Build history of the part. All positions in model axes, mm. Coordinates: 2 decimals unless noted, no trailing zeros. Loops run counter-clockwise (first coordinate to the right, second up) from the corner with the lowest first, then second, coordinate; pieces in that order, holes last. Notation, with made-up numbers: (21.5, 26.5) - (65.5, 26.5) arc R9 cw to (65.5, 40.5) - close; hole circle Ø7 at (-28, 86). An arc over 180 degrees is marked (long way). One line per item, written item: value.
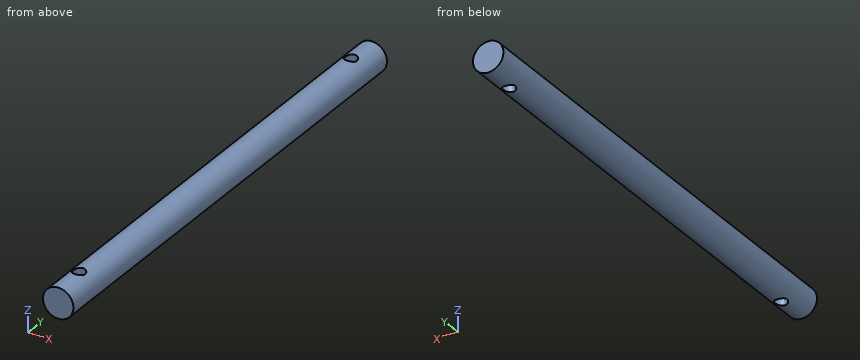
```python
from build123d import *

# Parameters (mm, degrees)
SKETCH1_R           = 3.96
BOSS_EXTRUDE1_DEPTH = 65.09
SKETCH2_R           = 1.59
CUT_EXTRUDE1_DEPTH  = 66.330477574


with BuildPart() as part:
    # Sketch1 → Boss-Extrude1 (new, symmetric)
    with BuildSketch(Plane(origin=(0, 0, 0), x_dir=(1, 0, 0), z_dir=(0, 1, 0))):
        with Locations(Location((0, 0, 0), (0, 0, 270))):
            Circle(SKETCH1_R)
    extrude(amount=BOSS_EXTRUDE1_DEPTH, both=True)

    # Sketch2 → Cut-Extrude1 (cut, symmetric)
    with BuildSketch(Plane.XY):
        with Locations(Location((0, 56.43, 0), (0, 0, 90))):
            Circle(SKETCH2_R)
    cut_extrude1 = extrude(amount=CUT_EXTRUDE1_DEPTH, both=True, mode=Mode.SUBTRACT)

    # Mirror1: Cut-Extrude1 across plane
    add(cut_extrude1.mirror(Plane.ZX), mode=Mode.SUBTRACT)


solid = part.part
```
Item 1: Cut at B-B, the plane z = 0. Write the cut outline in (x, y).
Check result:
outline: (-3.96, -65.09) - (3.96, -65.09) - (3.96, 65.09) - (-3.96, 65.09) - close; hole circle Ø3.18 at (0, -56.43); hole circle Ø3.18 at (0, 56.43)
Item 2: Cut at C-C, the plane y = 52. Write the cut outline in (x, z), then the cut area to 3 significant figures.
Check result:
outline: circle Ø7.92 at (0, 0)
area: 49.3 mm^2
Item 3: Probe probe 1 along Y at (x, z) = (0, -0.5); probe 2 along Y at (x, z) = (-1, -0.5); probe 3 along X at (y, z) = (47.5, 0.25). List the from-to ranges inside material, lowest first. Write a range as from..to.
Check result:
probe 1: y = -65.09..-58.02, -54.84..54.84, 58.02..65.09
probe 2: y = -65.09..-57.67, -55.19..55.19, 57.67..65.09
probe 3: x = -3.95..3.95
Item 4: Cut at A-A, the plane x = 0. Write the cut outline in (y, z), then the cut area to 3 significant figures.
Check result:
outline: (-65.09, -3.96) - (-58.02, -3.96) - (-58.02, 3.96) - (-65.09, 3.96) - close; (-54.84, -3.96) - (54.84, -3.96) - (54.84, 3.96) - (-54.84, 3.96) - close; (58.02, -3.96) - (65.09, -3.96) - (65.09, 3.96) - (58.02, 3.96) - close
area: 981 mm^2
Item 5: Drop flat-ended pins along their axis: P1, Ø4, axis at y = -37.5, z = 2.5, coming from the -X side; P2, Ø1, axis at x = 2.5, y = -28, coming from the -Z side; P3, Ø2, axis at y = 34.5, z = 2, coming from the -X side; P4, Ø4, axis at x = 0, y = -56.43, coming from the -Z side. Give the stop position or say it passes through.
Check result:
P1: stops at x = -3.93
P2: stops at z = -3.42
P3: stops at x = -3.83
P4: stops at z = -3.96
